The listing builds one solid part. Answer for the finished solid, in the listing's coordinates (mm). A direction names the side the tool comes from. Give positions to 0.01 mm unless a question says otherwise; leave off trailing zeros. Loops run counter-clockwise (first coordinate to the right, second up) from the corner with the lowest first, then second, coordinate; pieces in that order, holes last. Notation, with made-up numbers: M -2,10.5 L 51,10.5 A9 cw 51,16.5 Z; hole C 65,-20.75 d10. An arc over 180 degrees is marked long. One line per item, written item: value. Start each with the question number.
Q1. Flat-ended cylindrical pins translate along their axes: pin 1 (1 mm diameter, centred on x = -6, z = 18, fed in from -Y); pin 2 (8 mm diameter, centred on x = 7.5, y = 60.5, fed in from -Z); pin 3 (3 mm diameter, centred on x = -14, z = 4, fed in from -Y). Find the tip coordinate at first contact, or state that the pin passes through.
Q2. A cutting plane is placed at A-A, the plane y = 0. Determine the outline of the cut face in (x, z), and give its area (3 significant figures).
Q3. The mould has two halves that part along Y. Classify faces 3 (the flat face through (-0.11, 103.956, 21.588)), 4 (the flat face through (0, 35, 6)), 5 (the flat face through (-1, 9.2, 21.2)): +Y half, -Y half, draft (parallel to the pull), parting line (faces both ways), or undercut.
Q4. For faces 1 (the cylindrical face through (-1.02, 70.34, 7.87)), 2 (the cylindrical face through (11.71, 3.69, 20.19)), determine the directions among +Z, -Z, +X, -X, +Y, -Y from which every point of the face is accessible in a straight line to the end or side of a thin tool.
Q5. Consider L1, parallel to Y at x = 0, z = 14; L2, parallel to Z at x = 9, y = -3.5; L3, parallel to Y at x = 0, z = 15.75. Determine where each line is inside the solid, lowest interval first.
from build123d import *

# Parameters (mm, degrees)
SKETCH1_R               = 18
BOSS_EXTRUDE1_DEPTH     = 19.2
SKETCH2_R               = 12.276458432
SKETCH2_R_2             = 8.347690183
BOSS_EXTRUDE2_DEPTH     = 2
SKETCH3_R               = 8.347690183
BOSS_EXTRUDE4_DEPTH     = 6.8
FILLET1_R               = 4
SKETCH13_R              = 9
CUT_EXTRUDE4_DEPTH      = 50
BOSS_EXTRUDE6_START     = 36.124968835
BOSS_EXTRUDE6_OUTLINE_R = 7.85
BOSS_EXTRUDE6_DEPTH     = 70


with BuildPart() as part:
    # Sketch1 → Boss-Extrude1 (new body)
    with BuildSketch(Plane.XY):
        Circle(SKETCH1_R)
    extrude(amount=BOSS_EXTRUDE1_DEPTH)

    # Sketch2 → Boss-Extrude2 (add)
    with BuildSketch(Plane.XY.offset(19.2)):
        Circle(SKETCH2_R)
        Circle(SKETCH2_R_2, mode=Mode.SUBTRACT)
    extrude(amount=BOSS_EXTRUDE2_DEPTH)

    # Sketch3 → Boss-Extrude4 (add)
    with BuildSketch(Plane.XY.offset(19.2)):
        Circle(SKETCH3_R)
    extrude(amount=BOSS_EXTRUDE4_DEPTH)

    # Fillet1
    fillet1_edges = [part.edges().sort_by_distance(p)[0] for p in [
        (-8.347690183, 0, 26),
    ]]
    fillet(fillet1_edges, radius=FILLET1_R)

    # Loft5: read off the stored shape, not the designer's step
    # Loft5: loft between two sections, ruled curve by curve
    loft5_from = [
        Edge.make_bspline([(-13.870540046, 10, 1.272084055), (-13.870540046, 10, 2.733260237), (-13.870540046, 10, 4.19443642), (-13.870540046, 10, 7.116788785), (-13.870540046, 10, 8.577964967), (-13.870540046, 10, 11.500317332), (-13.870540046, 10, 12.961493515), (-13.870540046, 10, 15.88384588), (-13.870540046, 10, 17.345022062), (-13.870540046, 10, 18.806198245)], [0, 0, 0, 0, 0.25, 0.25, 0.5, 0.5, 0.75, 0.75, 1, 1, 1, 1], 3),
        Edge.make_bspline([(-13.870540046, 10, 18.806198245), (-12.638187033, 10, 18.806198245), (-11.40583402, 10, 18.806198245), (-8.941127993, 10, 18.806198245), (-7.70877498, 10, 18.806198245), (-5.244068953, 10, 18.806198245), (-4.01171594, 10, 18.806198245), (-1.547009913, 10, 18.806198245), (-0.3146569, 10, 18.806198245), (2.150049127, 10, 18.806198245), (3.38240214, 10, 18.806198245), (5.847108167, 10, 18.806198245), (7.07946118, 10, 18.806198245), (9.544167207, 10, 18.806198245), (10.77652022, 10, 18.806198245), (13.241226247, 10, 18.806198245), (14.47357926, 10, 18.806198245), (15.705932273, 10, 18.806198245)], [0, 0, 0, 0, 0.125, 0.125, 0.25, 0.25, 0.375, 0.375, 0.5, 0.5, 0.625, 0.625, 0.75, 0.75, 0.875, 0.875, 1, 1, 1, 1], 3),
        Edge.make_bspline([(15.293044741, 10, 1.272084055), (14.077895375, 10, 1.272084055), (12.862746008, 10, 1.272084055), (10.432447276, 10, 1.272084055), (9.21729791, 10, 1.272084055), (6.786999178, 10, 1.272084055), (5.571849812, 10, 1.272084055), (3.141551079, 10, 1.272084055), (1.926401713, 10, 1.272084055), (-0.503897019, 10, 1.272084055), (-1.719046385, 10, 1.272084055), (-4.149345117, 10, 1.272084055), (-5.364494484, 10, 1.272084055), (-7.794793216, 10, 1.272084055), (-9.009942582, 10, 1.272084055), (-11.440241314, 10, 1.272084055), (-12.65539068, 10, 1.272084055), (-13.870540046, 10, 1.272084055)], [0, 0, 0, 0, 0.125, 0.125, 0.25, 0.25, 0.375, 0.375, 0.5, 0.5, 0.625, 0.625, 0.75, 0.75, 0.875, 0.875, 1, 1, 1, 1], 3),
        Edge.make_bspline([(15.705932273, 10, 18.806198245), (15.671524979, 10, 17.345022062), (15.637117685, 10, 15.88384588), (15.568303096, 10, 12.961493515), (15.533895801, 10, 11.500317332), (15.465081213, 10, 8.577964967), (15.430673918, 10, 7.116788785), (15.361859329, 10, 4.19443642), (15.327452035, 10, 2.733260237), (15.293044741, 10, 1.272084055)], [0, 0, 0, 0, 0.25, 0.25, 0.5, 0.5, 0.75, 0.75, 1, 1, 1, 1], 3),
    ]
    loft5_to = [
        Edge.make_bspline([(-6.740203008, 35, 5.516591807), (-7.083985671, 35, 6.09243536), (-7.365341755, 35, 6.734156051), (-7.74869442, 35, 8.097700335), (-7.85, 35, 8.818869121), (-7.85, 35, 10.26221196), (-7.74869442, 35, 10.983380746), (-7.365341755, 35, 12.34692503), (-7.083985671, 35, 12.988645721), (-6.740203008, 35, 13.564489274)], [0, 0, 0, 0, 0.25, 0.25, 0.5, 0.5, 0.75, 0.75, 1, 1, 1, 1], 3),
        Edge.make_bspline([(-6.740203008, 35, 13.564489274), (-6.451756257, 35, 14.047643954), (-6.092847535, 35, 14.530224597), (-5.218696772, 35, 15.438416605), (-4.702923047, 35, 15.863536141), (-3.528860323, 35, 16.586454489), (-2.870504053, 35, 16.883315453), (-1.466341415, 35, 17.286893217), (-0.721281456, 35, 17.392785885), (0.769354223, 35, 17.388221597), (1.513751736, 35, 17.277768249), (2.915416578, 35, 16.865599114), (3.57194256, 35, 16.564712015), (4.741556195, 35, 15.834617391), (5.254716863, 35, 15.406347285), (6.123289567, 35, 14.492819102), (6.479236287, 35, 14.00804959), (6.764718843, 35, 13.523137554)], [0, 0, 0, 0, 0.125, 0.125, 0.25, 0.25, 0.375, 0.375, 0.5, 0.5, 0.625, 0.625, 0.75, 0.75, 0.875, 0.875, 1, 1, 1, 1], 3),
        Edge.make_bspline([(6.714912928, 35, 5.474529674), (6.424525906, 35, 4.994962936), (6.064332724, 35, 4.516631942), (5.189797582, 35, 3.61755227), (4.674946594, 35, 3.197289059), (3.505304255, 35, 2.483288448), (2.850457816, 35, 2.190459602), (1.45515568, 35, 1.792552317), (0.715425599, 35, 1.688265686), (-0.76450524, 35, 1.692892109), (-1.503568847, 35, 1.801801607), (-2.896355935, 35, 2.208424757), (-3.549358764, 35, 2.50534208), (-4.714514202, 35, 3.226641519), (-5.226727577, 35, 3.650115443), (-6.095624443, 35, 4.55464527), (-6.452819986, 35, 5.035218898), (-6.740203008, 35, 5.516591807)], [0, 0, 0, 0, 0.125, 0.125, 0.25, 0.25, 0.375, 0.375, 0.5, 0.5, 0.625, 0.625, 0.75, 0.75, 0.875, 0.875, 1, 1, 1, 1], 3),
        Edge.make_bspline([(6.764718843, 35, 13.523137554), (7.105005207, 35, 12.945137428), (7.382450639, 35, 12.301626641), (7.757449733, 35, 10.935584457), (7.854315981, 35, 10.21371246), (7.845383427, 35, 8.770216678), (7.739590849, 35, 8.049598762), (7.347714599, 35, 6.68830211), (7.062326449, 35, 6.048274216), (6.714912928, 35, 5.474529674)], [0, 0, 0, 0, 0.25, 0.25, 0.5, 0.5, 0.75, 0.75, 1, 1, 1, 1], 3),
    ]
    loft5 = Solid(Shell([*[Face.make_surface_from_curves(loft5_from[k], loft5_to[k]) for k in range(4)], Face(Wire(loft5_from)), Face(Wire(loft5_to))]))
    add(loft5)

    # Sketch13 → Cut-Extrude4 (cut)
    with BuildSketch(Plane(origin=(0, 0, 0), x_dir=(-1, 0, 0), z_dir=(0, 0, -1))):
        Circle(SKETCH13_R)
    extrude(amount=-CUT_EXTRUDE4_DEPTH, mode=Mode.SUBTRACT)


with BuildPart() as boss_extrude6_tool:
    # Boss-Extrude6: read off the stored shape, not the designer's step
    # Boss-Extrude6 outline → Boss-Extrude6 (new body)
    with BuildSketch(Plane(origin=(0, 0, 0), x_dir=(1, 0, 0), z_dir=(0, 0.9848077530122076, 0.1736481776669339)).offset(BOSS_EXTRUDE6_START)):
        with Locations((0, -3.317912074)):
            Circle(BOSS_EXTRUDE6_OUTLINE_R)
    extrude(amount=BOSS_EXTRUDE6_DEPTH)


with BuildPart() as part_1:
    add(part.part)


with BuildPart() as part_2:
    # Boss-Extrude6: joined with boss_extrude6_tool
    add(part_1.part.fuse(boss_extrude6_tool.part, tol=0.00001))


solid = part_2.part
Answer block:
1. pin 1: y = -17.14
1. pin 2: z = 6.79
1. pin 3: y = -12.95
2. outline: M -18,0 L -9,0 L -9,21.2 L -12.28,21.2 L -12.28,19.2 L -18,19.2 Z; M 9,0 L 18,0 L 18,19.2 L 12.28,19.2 L 12.28,21.2 L 9,21.2 Z
2. area: 359 mm^2
3. face 3: +Y half
3. face 4: undercut
3. face 5: draft
4. face 1: none
4. face 2: +Z
5. L1: -18 to -9, 9 to 105.29
5. L2: 0 to 21.2
5. L3: -18 to -9, 9 to 104.98
